CAD build for the part. Positions are in the model's coordinates, mm. A direction names the side the tool comes from. Round coordinates to 2 decimals unless told otherwise and drop trailing zeros. Loops run counter-clockwise (first coordinate to the right, second up) from the corner with the lowest first, then second, coordinate; pieces in that order, holes last.
from build123d import *

# Parameters (mm, degrees)
SKETCH1_R           = 52.5
BOSS_EXTRUDE1_DEPTH = 10


with BuildPart() as part:
    # Sketch1 → Boss-Extrude1 (new body)
    with BuildSketch(Plane.XY):
        Circle(SKETCH1_R)
        with BuildLine():
            ThreePointArc((38.40767043, -27.948181554), (23.75, -41.13620668), (5, -47.236109069))
            Line((5, -47.236109069), (5, -12))
            ThreePointArc((5, -12), (6.5, -11.258330249), (7.892304845, -10.330127019))
            Line((7.892304845, -10.330127019), (38.40767043, -27.948181554))
        make_face(mode=Mode.SUBTRACT)
        with BuildLine():
            ThreePointArc((-5, -47.236109069), (-23.75, -41.13620668), (-38.40767043, -27.948181554))
            Line((-38.40767043, -27.948181554), (-7.892304845, -10.330127019))
            ThreePointArc((-7.892304845, -10.330127019), (-6.5, -11.258330249), (-5, -12))
            Line((-5, -12), (-5, -47.236109069))
        make_face(mode=Mode.SUBTRACT)
        with BuildLine():
            Line((-1.658312395, 2.5), (1.658312395, 2.5))
            ThreePointArc((1.658312395, 2.5), (0, -3), (-1.658312395, 2.5))
        make_face(mode=Mode.SUBTRACT)
        with BuildLine():
            ThreePointArc((-43.40767043, -19.287927516), (-47.5, 0), (-43.40767043, 19.287927516))
            Line((-43.40767043, 19.287927516), (-12.892304845, 1.669872981))
            ThreePointArc((-12.892304845, 1.669872981), (-13, 0), (-12.892304845, -1.669872981))
            Line((-12.892304845, -1.669872981), (-43.40767043, -19.287927516))
        make_face(mode=Mode.SUBTRACT)
        with BuildLine():
            Line((-5, 47.236109069), (-5, 12))
            ThreePointArc((-5, 12), (-6.5, 11.258330249), (-7.892304845, 10.330127019))
            Line((-7.892304845, 10.330127019), (-38.40767043, 27.948181554))
            ThreePointArc((-38.40767043, 27.948181554), (-23.75, 41.13620668), (-5, 47.236109069))
        make_face(mode=Mode.SUBTRACT)
        with BuildLine():
            ThreePointArc((43.40767043, 19.287927516), (47.5, 0), (43.40767043, -19.287927516))
            Line((43.40767043, -19.287927516), (12.892304845, -1.669872981))
            ThreePointArc((12.892304845, -1.669872981), (13, 0), (12.892304845, 1.669872981))
            Line((12.892304845, 1.669872981), (43.40767043, 19.287927516))
        make_face(mode=Mode.SUBTRACT)
        with BuildLine():
            ThreePointArc((5, 47.236109069), (23.75, 41.13620668), (38.40767043, 27.948181554))
            Line((38.40767043, 27.948181554), (7.892304845, 10.330127019))
            ThreePointArc((7.892304845, 10.330127019), (6.5, 11.258330249), (5, 12))
            Line((5, 12), (5, 47.236109069))
        make_face(mode=Mode.SUBTRACT)
    extrude(amount=BOSS_EXTRUDE1_DEPTH)


solid = part.part
Item 1: Flat gauge pins, fed straight in: P1, Ø1.5, axis at y = 34.5, z = 4.5, coming from the +X side; P2, Ø4, axis at x = 36, z = 9, coming from the +Y side; P3, Ø3.5, axis at x = -0.5, z = 5.5, coming from the -Y side. Where does each tip first touch, or does it go through?
Verdict:
P1: stops at x = 40.21
P2: stops at y = 40
P3: stops at y = -52.5
Item 2: Cut at D-D (x = 33.5). List the corners of the cut face in (y, z).
Verdict:
outline: (-40.42, 0) - (-33.67, 0) - (-33.67, 10) - (-40.42, 10) - close; (-25.11, 0) - (-13.57, 0) - (-13.57, 10) - (-25.11, 10) - close; (13.57, 0) - (25.11, 0) - (25.11, 10) - (13.57, 10) - close; (33.67, 0) - (40.42, 0) - (40.42, 10) - (33.67, 10) - close
Item 3: Cut at C-C (y = 0). List the corners of the cut face in (x, z), plus the area to 3 significant figures.
Verdict:
outline: (-52.5, 0) - (-47.5, 0) - (-47.5, 10) - (-52.5, 10) - close; (-13, 0) - (-3, 0) - (-3, 10) - (-13, 10) - close; (3, 0) - (13, 0) - (13, 10) - (3, 10) - close; (47.5, 0) - (52.5, 0) - (52.5, 10) - (47.5, 10) - close
area: 300 mm2
Item 4: Cut at B-B (x = 0). List the corners of the cut face in (y, z).
Verdict:
outline: (-52.5, 0) - (-3, 0) - (-3, 10) - (-52.5, 10) - close; (2.5, 0) - (52.5, 0) - (52.5, 10) - (2.5, 10) - close
Item 5: Wall check: L1, parallel to X at y = -22.5, z = 3; L2, parallel to Y at x = 0, z = 7.75; L3, parallel to X at y = -43, z = 3.75. Give the ranges that are in metal, low to high.
Verdict:
L1: x = -47.43 to -28.97, -5 to 5, 28.97 to 47.43
L2: y = -52.5 to -3, 2.5 to 52.5
L3: x = -30.12 to -20.18, -5 to 5, 20.18 to 30.12
Item 6: Cut at A-A (z = 8.5). List the corners of the cut face in (x, y).
Verdict:
outline: circle Ø105 at (0, 0); hole (-43.41, -19.29) - (-12.89, -1.67) arc R13 cw to (-12.89, 1.67) - (-43.41, 19.29) arc R47.5 ccw to start; hole (-38.41, -27.95) arc R47.5 ccw to (-5, -47.24) - (-5, -12) arc R13 cw to (-7.89, -10.33) - close; hole (-38.41, 27.95) - (-7.89, 10.33) arc R13 cw to (-5, 12) - (-5, 47.24) arc R47.5 ccw to start; hole (-1.66, 2.5) arc R3 ccw (long way) to (1.66, 2.5) - close; hole (5, -47.24) arc R47.5 ccw to (38.41, -27.95) - (7.89, -10.33) arc R13 cw to (5, -12) - close; hole (5, 12) arc R13 cw to (7.89, 10.33) - (38.41, 27.95) arc R47.5 ccw to (5, 47.24) - close; hole (12.89, -1.67) - (43.41, -19.29) arc R47.5 ccw to (43.41, 19.29) - (12.89, 1.67) arc R13 cw to start
Item 7: 3-axis set-ups, long thin cutter, end or side, ignore diameter. For faces 1 (the cylindrical face through (6.48, -11.27, 4.93)), 2 (the flat face through (-1, -11, 0)): which of +Z, -Z, +X, -X, +Y, -Y reach the whole face in a straight line?
Verdict:
face 1: +Z, -Z
face 2: -Z, +X, -X, +Y, -Y
